Model file for the job. Use its own axes, mm. A direction names the side the tool comes from. Round coordinates to 2 decimals unless told otherwise and drop trailing zeros. Write each loop counter-clockwise with the first axis right and the second up, starting at its lowest first coordinate (ties: lowest second). Pieces come first, ordered by that corner, then holes.
```python
from build123d import *

# Parameters (mm, degrees)
F0_R     = 144.070975
F1_DEPTH = 172
F2_W     = 137.853176
F2_H     = 141.037912
F3_DEPTH = 25
F4_R     = 48.783295
F5_DEPTH = 94
F6_R     = 71.562045
F6_R_2   = 60.159881
F7_DEPTH = 19


with BuildPart() as f1:
    # F0 (on Front) → F1 (new body)
    with BuildSketch(Plane.XZ):
        Circle(F0_R)
    extrude(amount=F1_DEPTH)

    # F2 (on face) → F3 (join)
    with BuildSketch(Plane.XZ.offset(172)):
        Rectangle(F2_W, F2_H)
    extrude(amount=F3_DEPTH)

    # F4 (on face) → F5 (join)
    with BuildSketch(Plane.XZ.offset(197)):
        Circle(F4_R)
    extrude(amount=F5_DEPTH)

    # F6 (on Right) → F7 (join, symmetric)
    with BuildSketch(Plane.YZ):
        with Locations((-358.792186, 0)):
            Circle(F6_R)
        with Locations((-358.792186, 0)):
            Circle(F6_R_2, mode=Mode.SUBTRACT)
    extrude(amount=F7_DEPTH, both=True)


solid = f1.part
```
1) Wall check: probe 1 along Y at (x, z) = (-73, -59); probe 2 along X at (y, z) = (-390, -54); probe 3 along Y at (x, z) = (60.5, -11). Give the ranges that are in metal, low to high.
2) Flat gauge pins, fed straight in: pin 1 Ø4 at (x, z) = (-74, -67) entering from -Y; pin 2 Ø20 at (y, z) = (-184.5, -22.5) entering from -X; pin 3 Ø10 at (y, z) = (-97.5, 94) entering from +X. Where does each tip first touch, or does it go through?
3) Cut at C-C on y = -389. List the corners of the cut face in (x, z), and give its area (3 significant figures).
4) Which spindle directions (+Z, -Z, +X, -X, +Y, -Y) get a long thin tool onto all of the face, cutting with end or side? Do faces 1 (the face through (-1, -184, 70.519)), 2 (the face through (68.927, -184, -1)), 3 (the face through (21, -291, 1)). Say none if no direction does.
5) Cut at A-A on z = 0. List the corners of the cut face in (x, y), and give its area (3 significant figures).
6) Cut at B-B on z = -35.5. List the corners of the cut face in (x, y).
7) Cut at D-D on x = 4. List the corners of the cut face in (y, z).
8) Pull direction Y, two halves, no side cores. Call faces 4 (the face through (-2, 0, 2)), 5 (the face through (-35.955, -243.342, 32.97)), 6 (the face through (-19, -402.3, -42.1)): released by +Y, released by -Y, zero draft, split by the parting line, or undercut.
Result sheet:
1. probe 1: y = -172 to 0
1. probe 2: x = -19 to 19
1. probe 3: y = -197 to 0
2. pin 1: stops at y = -172
2. pin 2: stops at x = -68.93
2. pin 3: stops at x = 113.29
3. outline: (-19, -64.87) - (19, -64.87) - (19, -52.03) - (-19, -52.03) - close; (-19, 52.03) - (19, 52.03) - (19, 64.87) - (-19, 64.87) - close
3. area: 976 mm2
4. face 1: +Z, +X, -X
4. face 2: +Z, -Z, +X, -Y
4. face 3: none
5. outline: (-144.07, -172) - (-68.93, -172) - (-68.93, -197) - (-48.78, -197) - (-48.78, -291) - (-19, -291) - (-19, -298.63) - (19, -298.63) - (19, -291) - (48.78, -291) - (48.78, -197) - (68.93, -197) - (68.93, -172) - (144.07, -172) - (144.07, 0) - (-144.07, 0) - close; (-19, -430.35) - (19, -430.35) - (19, -418.95) - (-19, -418.95) - close
5. area: 62,900 mm2
6. outline: (-139.63, -172) - (-68.93, -172) - (-68.93, -197) - (-33.46, -197) - (-33.46, -291) - (33.46, -291) - (33.46, -197) - (68.93, -197) - (68.93, -172) - (139.63, -172) - (139.63, 0) - (-139.63, 0) - close; (-19, -420.93) - (19, -420.93) - (19, -407.36) - (-19, -407.36) - close; (-19, -310.22) - (19, -310.22) - (19, -296.66) - (-19, -296.66) - close
7. outline: (-291, -48.62) - (-197, -48.62) - (-197, -70.52) - (-172, -70.52) - (-172, -144.02) - (0, -144.02) - (0, 144.02) - (-172, 144.02) - (-172, 70.52) - (-197, 70.52) - (-197, 48.62) - (-291, 48.62) - (-291, 22.92) arc R71.56 ccw (long way) to (-291, -22.92) - close; hole circle Ø120.32 at (-358.79, 0)
8. face 4: released by +Y
8. face 5: undercut
8. face 6: zero draft
